Source: CAD feature listing. Evaluate the final solid. Frame: model axes, mm. Face numbers are marked on the shaded views. A direction names the side the tool comes from. Round coordinates to 2 decimals unless told otherwise and drop trailing zeros. Loops run counter-clockwise (first coordinate to the right, second up) from the corner with the lowest first, then second, coordinate; pieces in that order, holes last. Notation, with made-up numbers: (27, 30) -> (64, 30) arc R10 ccw to (64, 40) -> close; hole circle Ø1 at (42, -20). An arc over 180 degrees is marked (long way). Write item = value, one per line.
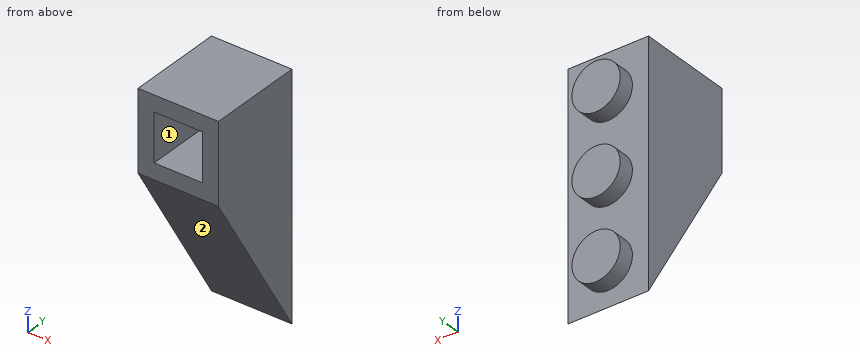
from build123d import *

# Parameters (mm, degrees)
SKETCH1_W           = 8
SKETCH1_H           = 9.6
BOSS_EXTRUDE1_DEPTH = 8
SHELL2_T            = -1.6
BOSS_EXTRUDE3_DEPTH = 8
SKETCH4_R           = 2.4
BOSS_EXTRUDE4_DEPTH = 1.6
LPATTERN2_COUNT     = 3
LPATTERN2_PITCH     = 8


with BuildPart() as part:
    # Sketch1 → Boss-Extrude1 (new body)
    with BuildSketch(Plane(origin=(0, 0, 0), x_dir=(0, 0, -1), z_dir=(1, 0, 0))):
        with Locations((4, 4.8)):
            Rectangle(SKETCH1_W, SKETCH1_H)
    extrude(amount=BOSS_EXTRUDE1_DEPTH)

    # Shell2
    shell2_openings = [part.faces().sort_by_distance(p)[0] for p in [
        (4, 0, -4),
    ]]
    offset(amount=SHELL2_T, openings=shell2_openings, kind=Kind.INTERSECTION)

    # Sketch3 → Boss-Extrude3 (add)
    with BuildSketch(Plane(origin=(0, 0, 0), x_dir=(0, 0, -1), z_dir=(1, 0, 0))):
        Polygon((8, 0), (24, 9.6), (8, 9.6), align=None)
    extrude(amount=BOSS_EXTRUDE3_DEPTH)

    # Sketch4 → Boss-Extrude4 (add)
    with BuildSketch(Plane(origin=(0, 9.6, 0), x_dir=(1, 0, 0), z_dir=(0, 1, 0))):
        with Locations(Location((4, 4, 0), (0, 0, 90))):
            Circle(SKETCH4_R)
    boss_extrude4 = extrude(amount=BOSS_EXTRUDE4_DEPTH)

    # LPattern2: Boss-Extrude4 ×3
    with Locations(*[(0, 0, -i * LPATTERN2_PITCH) for i in range(1, LPATTERN2_COUNT)]):
        add(boss_extrude4)


solid = part.part
1. Section query B-B (z = -20). Return the cut outline in (x, y), then the cut area to 3 significant figures.
Evaluation:
outline = (0, 7.2) -> (8, 7.2) -> (8, 9.6) -> (6.4, 9.6) -> (6.4, 11.2) -> (1.6, 11.2) -> (1.6, 9.6) -> (0, 9.6) -> close
area = 26.9 mm²
2. Line query: probe 1 along X at (y, z) = (3.25, -6); probe 2 along Y at (x, z) = (1.75, -3); probe 3 along Z at (x, y) = (5.5, 10.75). Output: solid intervals per line, ascending. Write a range as from..to.
Evaluation:
probe_1 = 0..1.6, 6.4..8
probe_2 = 8..9.6
probe_3 = -21.87..-18.13, -13.87..-10.13, -5.87..-2.13
3. Section query D-D (y = 3). Return the cut outline in (x, z).
Evaluation:
outline = (0, -13) -> (8, -13) -> (8, 0) -> (0, 0) -> close; hole (1.6, -6.4) -> (6.4, -6.4) -> (6.4, -1.6) -> (1.6, -1.6) -> close
4. Section query A-A (y = 6.75). Return the cut outline in (x, z), then the cut area to 3 significant figures.
Evaluation:
outline = (0, -19.25) -> (8, -19.25) -> (8, 0) -> (0, 0) -> close; hole (1.6, -6.4) -> (6.4, -6.4) -> (6.4, -1.6) -> (1.6, -1.6) -> close
area = 131 mm²
5. Contact query for flat-ended pins moving along their axis: pin 1 Ø1.5 at (y, z) = (5.5, -20) entering from +X; pin 2 Ø3 at (x, z) = (2, -11.5) entering from -Y; pin 3 Ø1 at (x, z) = (4, -9) entering from -Y; pin 4 Ø1.4 at (x, z) = (4.5, -4) entering from -Y. Output: stop coordinate, or through.
Evaluation:
pin_1 = through
pin_2 = 1.2
pin_3 = 0.3
pin_4 = 8
6. Section query C-C (x = 4). Return the cut outline in (y, z).
Evaluation:
outline = (0, -8) -> (9.6, -24) -> (9.6, -22.4) -> (11.2, -22.4) -> (11.2, -17.6) -> (9.6, -17.6) -> (9.6, -14.4) -> (11.2, -14.4) -> (11.2, -9.6) -> (9.6, -9.6) -> (9.6, -6.4) -> (11.2, -6.4) -> (11.2, -1.6) -> (9.6, -1.6) -> (9.6, 0) -> (0, 0) -> (0, -1.6) -> (8, -1.6) -> (8, -6.4) -> (0, -6.4) -> close
7. Set-up query: the marked faces 1 and 2. Return all of +Z, -Z, +X, -X, +Y, -Y with unobstructed straight access to the full face (end or side cutting, diameter ignored); none if empty.
Evaluation:
face_1 = -Y
face_2 = -Z, +X, -X, -Y
